Design review of the part built by this model. Coordinates are the model's own, in mm. Face numbers are marked on the shaded views. A direction names the side the tool comes from. Coordinates: 2 decimals unless noted, no trailing zeros. Write each loop counter-clockwise with the first axis right and the second up, starting at its lowest first coordinate (ties: lowest second). Pieces come first, ordered by that corner, then holes.
Autodesk Inventor part; units mm, degrees
ref_plane "Start Plane" through (0, 0, 0) normal (1, 0, 0) x (0, 1, 0)
ref_plane "XZ Plane" through (0, 0, 0) normal (0, 1, 0) x (-1, 0, 0)
ref_plane "XY Plane" through (0, 0, 0) normal (0, 0, 1) x (1, 0, 0)
sketch "Main Sketch" plane through (0, 0, 0) normal (0, 0, 1) x (1, 0, 0)
  line L0 (0, 0) -> (123, 0)
  line L1 (0, 0) -> (0, 12.5)
  line L2 (0, 12.5) -> (60, 12.5)
  line L3 (60, 12.5) -> (60, 17.5)
  line L4 (63, 17.5) -> (63, 12.5)
  line L5 (60, 17.5) -> (63, 17.5)
  line L6 (123, 12.5) -> (123, 0)
  line L7 (63, 12.5) -> (123, 12.5)
  dimension "d3" = 25
  dimension "d4" = 35
  dimension "d5" = 25
revolve "Revolution1" add sketch "Main Sketch" angle 360 about axis through (0, 0, 0) along (1, 0, 0)
chamfer "Chamfer3" distance 0.5 angle 45 1 edges at (60, -17.5, 0) measured on face at (62, 17.4433, -1.4082)
fillet "Fillet2" radius 2 1 edges at (63, -17.5, 0)
chamfer "Chamfer4" distance 0.5 angle 45 1 edges at (63, -12.5, 0) measured on face at (103, 12.4595, -1.0058)
fillet "Fillet3" radius 2 1 edges at (123, -12.5, 0)
chamfer "Chamfer1" distance 0.5 angle 45 1 edges at (0, -12.5, 0) measured on face at (40, 12.4595, -1.0058)
fillet "Fillet1" radius 5 1 edges at (60, -12.5, 0)
equation "\"Length\" = 123"
properties part number "Shaft" material "Steel"
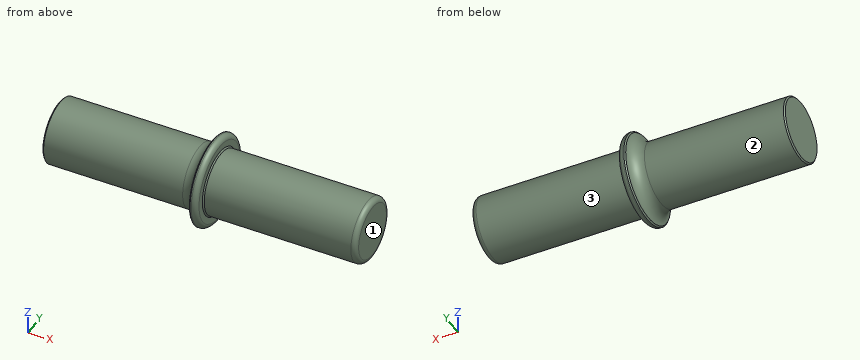
(1) Insertion check: pin 1 Ø3 at (x, y) = (68, -12) entering from -Z; pin 2 Ø1 at (x, z) = (36, -8.5) entering from -Y; pin 3 Ø1.5 at (x, z) = (81, -12) entering from -Y. Each pin has a flat end and moves straight along its axis. Give the tip position at first contact, or say it passes through.
(2) Consider section C-C (x = 67). Give the boundary of the cut face in (y, z), plus the area to 3 significant figures.
(3) For the marked faces 1, 2 and 3, list the 3-axis set-ups (+Z, -Z, +X, -X, +Y, -Y) from which the entire face can be reached by the end or side of a thin tool; tool diameter is ignored.
(4) Consider section A-A (z = 0). Give the boundary of the cut face in (x, y), plus the area to 3 significant figures.
(5) Wall thickness on line 1 (Y direction, x = 57, z = 7.5); line 2 (Z direction, x = 48, y = 0); line 3 (Z direction, x = 58.5, y = 7): over which ranges is each line inside the solid? List them lowest first.
Results:
1. pin 1: stops at z = -6.78
1. pin 2: stops at y = -9.6
1. pin 3: stops at y = -5.45
2. outline: circle Ø25 at (0, 0)
2. area: 491 mm2
3. face 1: +Z, -Z, +X, +Y, -Y
3. face 2: -X
3. face 3: +X
4. outline: (0, -12) - (0.5, -12.5) - (55.03, -12.5) arc R5 cw to (60, -17) - (60.5, -17.5) - (61, -17.5) arc R2 ccw to (63, -15.5) - (63, -13) - (63.5, -12.5) - (121, -12.5) arc R2 ccw to (123, -10.5) - (123, 10.5) arc R2 ccw to (121, 12.5) - (63.5, 12.5) - (63, 13) - (63, 15.5) arc R2 ccw to (61, 17.5) - (60.5, 17.5) - (60, 17) arc R5 cw to (55.03, 12.5) - (0.5, 12.5) - (0, 12) - close
4. area: 3,110 mm2
5. line 1: y = -10.5 to 10.5
5. line 2: z = -12.5 to 12.5
5. line 3: z = -12.01 to 12.01
